```python
from build123d import *

# Parameters (mm, degrees)
SKETCH1_R           = 5.08
SKETCH1_R_2         = 12.7
BOSS_EXTRUDE1_DEPTH = 5
SKETCH2_R           = 15.7
SKETCH2_R_2         = 12.7
BOSS_EXTRUDE2_DEPTH = 150


with BuildPart() as part:
    # Sketch1 → Boss-Extrude1 (new body)
    with BuildSketch(Plane.XY):
        with BuildLine():
            Line((17.630429803, 6.515946667), (8.338716799, 31.656866667))
            ThreePointArc((8.338716799, 31.656866667), (0, 37.465), (-8.338716799, 31.656866667))
            Line((-8.338716799, 31.656866667), (-17.630429803, 6.515946667))
            ThreePointArc((-17.630429803, 6.515946667), (-18.796, 0), (-17.630429803, -6.515946667))
            Line((-17.630429803, -6.515946667), (-8.338716799, -31.656866667))
            ThreePointArc((-8.338716799, -31.656866667), (0, -37.465), (8.338716799, -31.656866667))
            Line((8.338716799, -31.656866667), (17.630429803, -6.515946667))
            ThreePointArc((17.630429803, -6.515946667), (18.796, 0), (17.630429803, 6.515946667))
        make_face()
        with Locations((0, 28.575)):
            Circle(SKETCH1_R, mode=Mode.SUBTRACT)
        Circle(SKETCH1_R_2, mode=Mode.SUBTRACT)
        with Locations((0, -28.575)):
            Circle(SKETCH1_R, mode=Mode.SUBTRACT)
    extrude(amount=-BOSS_EXTRUDE1_DEPTH)

    # Sketch2 → Boss-Extrude2 (add)
    with BuildSketch(Plane.XY):
        Circle(SKETCH2_R)
        Circle(SKETCH2_R_2, mode=Mode.SUBTRACT)
    extrude(amount=-BOSS_EXTRUDE2_DEPTH)


solid = part.part
```
Can you work these out from the model? Positions are in its coordinate system, mm. A direction names the side the tool comes from. Give positions to 0.01 mm unless a question says otherwise; leave off trailing zeros. Loops run counter-clockwise (first coordinate to the right, second up) from the corner with the lowest first, then second, coordinate; pieces in that order, holes last. Notation, with made-up numbers: M 45.25,-28 L 68.25,-28 A28 ccw 68.25,-1 Z; hole C 56.5,6 d6. An arc over 180 degrees is marked long. One line per question, with ' | ' between items. Start each with the question number.
Q1. If I drill on line 1 (Y direction, x = 0, z = -86.5); line 2 (Y direction, x = -9, z = -93.5); line 3 (X direction, y = -6, z = -12), over which ranges is the centre line in solid material (lowest first)? Write a range as from..to.
Q2. For faces 1 (the cylindrical face through (-11.57, 10.61, -76.48)), 2 (the cylindrical face through (-0.151, -37.464, -2.465)), which set-ups out of +Z, -Z, +X, -X, +Y, -Y let a thin tool reach every point of the face, with its end or its side?
Q3. If we mould it in two halves opening along X, with no side actions, what happens to faces 3 (the flat face through (16, 1, -5)), 4 (the cylindrical face through (-18.796, 0.093, -2.465)), 5 (the cylindrical face through (-1.101, -33.534, -2.465)), 6 (the cylindrical face through (-2.75, -12.4, -73.95))? For each: +X half, -X half, draft (parallel to the pull), parting line (faces both ways), or undercut.
Q4. If we section it at C-C (x = -10.5): Please give me the cut outline in (y, z).
Q5. If we section it at B-B (y = 0): Please give me the cut outline in (x, z).
Q6. If we section it at D-D (z = -68.5): Please give me the cut outline in (x, y).
Q7. For pin 1 Ø2 at (y, z) = (3.5, -87) entering from -X; pin 2 Ø12 at (x, z) = (12, -52.5) entering from -Y; pin 3 Ø6 at (x, z) = (-7.5, -29) entering from +Y, each with a flat end and sliding along its axis, tell me the tip position at first contact or that it passes through.
Q8. If we section it at A-A (x = 0): Please give me the cut outline in (y, z) (3 decimals).
Computed:
1) line 1: y = -15.7..-12.7, 12.7..15.7 | line 2: y = -12.86..-8.96, 8.96..12.86 | line 3: x = -14.51..-11.19, 11.19..14.51
2) face 1: -Z | face 2: +Z, -Z, -Y
3) face 3: draft | face 4: -X half | face 5: undercut | face 6: undercut
4) outline: M -25.81,-5 L -11.67,-5 L -11.67,-150 L -7.14,-150 L -7.14,0 L -25.81,0 Z; M 7.14,-150 L 11.67,-150 L 11.67,-5 L 25.81,-5 L 25.81,0 L 7.14,0 Z
5) outline: M -18.8,-5 L -15.7,-5 L -15.7,-150 L -12.7,-150 L -12.7,0 L -18.8,0 Z; M 12.7,-150 L 15.7,-150 L 15.7,-5 L 18.8,-5 L 18.8,0 L 12.7,0 Z
6) outline: C 0,0 d31.4; hole C 0,0 d25.4
7) pin 1: stops at x = -15.5 | pin 2: stops at y = -14.51 | pin 3: stops at y = 15.04
8) outline: M -37.465,-5 L -33.655,-5 L -33.655,0 L -37.465,0 Z; M -23.495,-5 L -15.7,-5 L -15.7,-150 L -12.7,-150 L -12.7,0 L -23.495,0 Z; M 12.7,-150 L 15.7,-150 L 15.7,-5 L 23.495,-5 L 23.495,0 L 12.7,0 Z; M 33.655,-5 L 37.465,-5 L 37.465,0 L 33.655,0 Z
